Input: dimensioned drawing with shaded views. Units: mm. Origin: part minimum x, y, z. Round coordinates to 2 decimals unless told otherwise and drop trailing zeros. Write each loop counter-clockwise with the first axis right and the second up, starting at its lowest first coordinate (ties: lowest second). Pieces come first, ordered by that corner, then holes. Notation, with made-up numbers: M 85.25,39.5 L 89.25,39.5 A33 cw 89.25,77.5 Z; hole C 66.25,83 d6. An arc over 180 degrees is marked long. Answer as CSV lines item,"result". Start each with the question number.
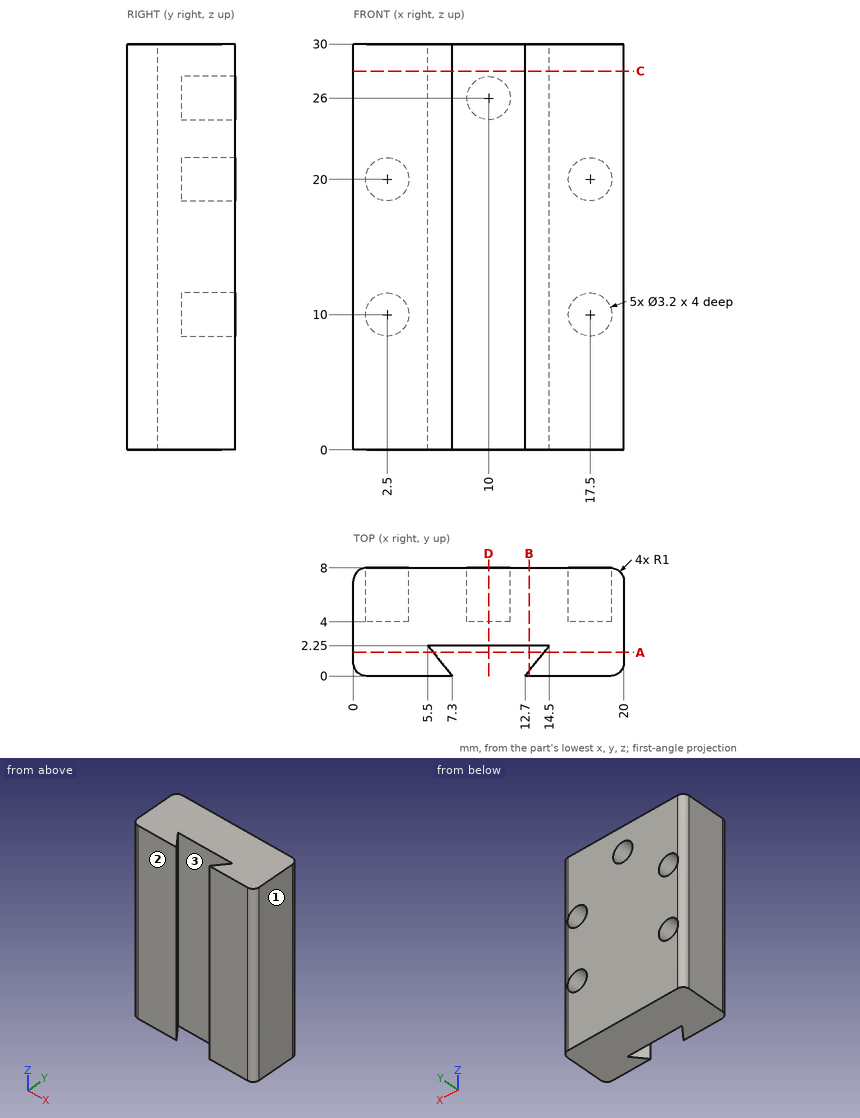
Item 1: Pin query (flat end, axial travel): pin 1 Ø1.6 at (x, z) = (2.5, 19.5) entering from +Y; pin 2 Ø5 at (x, z) = (10, 26) entering from +Y. Return the tip coordinate at first contact, or that it passes through.
Item 2: Line query: line 1 (X direction, y = 6.6, z = 20); line 2 (X direction, y = 4.9, z = 26); line 3 (X direction, y = 7, z = 20.5). Output: solid intervals per line, ascending. Write a range as [from, to].
Item 3: Cut plane A-A, the plane y = 1.75. Return loops of the section in (x, z), plus the area to 3 significant figures.
Item 4: Cut plane B-B, the plane x = 13. Return loops of the section in (y, z) (3 decimals).
Item 5: Cut plane C-C, the plane z = 28. Return loops of the section in (x, y).
Item 6: Cut plane D-D, the plane x = 10. Return loops of the section in (y, z).
Item 7: Draft query along X for the marked faces 1, 2 and 3. Return one class per face: +X half, -X half, draft (parallel to the pull), parting line (faces both ways), or undercut.
Results list:
1,pin 1,"y = 4"
1,pin 2,"y = 8"
2,line 1,"[0, 0.9], [4.1, 15.9], [19.1, 20]"
2,line 2,"[0, 8.4], [11.6, 20]"
2,line 3,"[0, 0.98], [4.02, 15.98], [19.02, 20]"
3,outline,"M 0,0 L 5.9,0 L 5.9,30 L 0,30 Z; M 14.1,0 L 20,0 L 20,30 L 14.1,30 Z"
3,area,"354 mm²"
4,outline,"M 0,0 L 0.375,0 L 0.375,30 L 0,30 Z; M 2.25,0 L 8,0 L 8,30 L 2.25,30 Z"
5,outline,"M 0,1 A1 ccw 1,0 L 7.3,0 L 5.5,2.25 L 14.5,2.25 L 12.7,0 L 19,0 A1 ccw 20,1 L 20,7 A1 ccw 19,8 L 1,8 A1 ccw 0,7 Z"
6,outline,"M 2.25,0 L 8,0 L 8,24.4 L 4,24.4 L 4,27.6 L 8,27.6 L 8,30 L 2.25,30 Z"
7,face 1,"+X half"
7,face 2,"draft"
7,face 3,"undercut"
